```python
from build123d import *

# Parameters (mm, degrees)
F1_DEPTH = 12
F2_R     = 1.1
F3_DEPTH = 6.5
F4_R     = 2.5
F5_DEPTH = 25
F7_DEPTH = 32


with BuildPart() as f1:
    # F0 (on Right) → F1 (new body)
    with BuildSketch(Plane.YZ):
        Polygon((35.1, -0.075058), (-4.9, -0.075058), (-4.9, -25.075058), (0, -25.075058), (0, -10.075058), (3.1, -10.075058), (3.1, -25.075058), (35.1, -25.075058), align=None)
    extrude(amount=F1_DEPTH)

    # F2 (on face) → F3 (cut)
    with BuildSketch(Plane.YZ.offset(12)):
        Polygon((34.6, -2.396713), (18.6, -2.396713), (18.6, -22.896713), (34.6, -22.896713), (34.6, -13.396713), (38.479045, -13.396713), (38.479045, -2.396713), align=None)
        with Locations((26.6, -17.646713)):
            Circle(F2_R, mode=Mode.SUBTRACT)
        with Locations((26.6, -7.646713)):
            Circle(F2_R, mode=Mode.SUBTRACT)
    extrude(amount=-F3_DEPTH, mode=Mode.SUBTRACT)

    # F4 (on face) → F5 (cut)
    with BuildSketch(Plane(origin=(0, 18.6, 0), x_dir=(-1, 0, 0), z_dir=(0, 1, 0))):
        with Locations((-8.783709, -5.351877)):
            Circle(F4_R)
    extrude(amount=-F5_DEPTH, mode=Mode.SUBTRACT)

    # F6 (on face) → F7 (cut, through all)
    with BuildSketch(Plane(origin=(0, 35.1, 0), x_dir=(-1, 0, 0), z_dir=(0, 1, 0))):
        Polygon((1.341271, -20.075058), (-0.25, -20.075058), (-2.75, -22.575058), (-2.75, -25.075058), (1.341271, -25.075058), align=None)
    extrude(amount=-F7_DEPTH, mode=Mode.SUBTRACT)


solid = f1.part
```
Geometry check sheet. Reference: the model listing, model coordinates, mm. A direction names the side the tool comes from. Coordinates: 2 decimals unless noted, no trailing zeros. Loops run counter-clockwise (first coordinate to the right, second up) from the corner with the lowest first, then second, coordinate; pieces in that order, holes last. Notation, with made-up numbers: (29.5, 10.5) -> (80.5, 10.5) arc R33 ccw to (80.5, 46.5) -> close; hole circle Ø11 at (78, -5.5). An arc over 180 degrees is marked (long way). Put each result on its own line as item: value.
1) Gauge pin test, flat ends, axial feed: pin 1 Ø4 at (x, z) = (8.78, -5.35) entering from +Y; pin 2 Ø1.2 at (y, z) = (21.5, -24) entering from -X; pin 3 Ø1.6 at (x, y) = (4.5, 1.5) entering from -Z. Record the tip position at first contact, or that the pin passes through.
Result set:
pin 1: stops at y = 27.66
pin 2: stops at x = 2.75
pin 3: stops at z = -10.08
2) Release check for a two-part mould opening along X. For faces 4 (the cylindrical face through (6.4, 7, -4.6)), 5 (the flat face through (12, 10, -12)), 6 (the cylindrical face through (8.8, 27.19, -16.72)) record: released by +X, released by -X, zero draft, split by the parting line, or undercut.
Result set:
face 4: undercut
face 5: released by +X
face 6: zero draft
3) Cross-section at A-A on z = -15.5. Record the boundary of the cut face in (x, y), plus the area to 3 significant figures.
Result set:
outline: (0, -4.9) -> (12, -4.9) -> (12, 0) -> (0, 0) -> close; (0, 3.1) -> (12, 3.1) -> (12, 18.6) -> (5.5, 18.6) -> (5.5, 34.6) -> (12, 34.6) -> (12, 35.1) -> (0, 35.1) -> close
area: 339 mm^2
4) Tool access check on faces 1 (the flat face through (9, 34.6, -18)), 2 (the flat face through (6, 3.1, -17)), 3 (the flat face through (1.483, 19.324, -21.308)). Record the directions out of +Z, -Z, +X, -X, +Y, -Y that give a thin tool (end or side, any length) a straight path to the whole face; none if there is none.
Result set:
face 1: +X
face 2: -Z, +X, -X
face 3: -Z, -X, +Y
5) Cross-section at D-D on z = -12.5. Record the boundary of the cut face in (x, y).
Result set:
outline: (0, -4.9) -> (12, -4.9) -> (12, 0) -> (0, 0) -> close; (0, 3.1) -> (12, 3.1) -> (12, 18.6) -> (5.5, 18.6) -> (5.5, 35.1) -> (0, 35.1) -> close
6) Cross-section at C-C on y = 26.6. Record the boundary of the cut face in (x, z).
Result set:
outline: (0, -20.08) -> (0.25, -20.08) -> (2.75, -22.58) -> (2.75, -25.08) -> (12, -25.08) -> (12, -22.9) -> (5.5, -22.9) -> (5.5, -18.75) -> (12, -18.75) -> (12, -16.55) -> (5.5, -16.55) -> (5.5, -8.75) -> (12, -8.75) -> (12, -6.55) -> (5.5, -6.55) -> (5.5, -2.4) -> (12, -2.4) -> (12, -0.08) -> (0, -0.08) -> close
7) Cross-section at B-B on x = 9. Record the boundary of the cut face in (y, z), plus the area to 3 significant figures.
Result set:
outline: (-4.9, -25.08) -> (0, -25.08) -> (0, -10.08) -> (3.1, -10.08) -> (3.1, -25.08) -> (35.1, -25.08) -> (35.1, -13.4) -> (34.6, -13.4) -> (34.6, -22.9) -> (18.6, -22.9) -> (18.6, -7.84) -> (-4.9, -7.84) -> close; (-4.9, -2.86) -> (18.6, -2.86) -> (18.6, -2.4) -> (35.1, -2.4) -> (35.1, -0.08) -> (-4.9, -0.08) -> close; circle Ø2.2 at (26.6, -17.65); circle Ø2.2 at (26.6, -7.65)
area: 511 mm^2
8) Thickness scan on line 1 (Y direction, x = 8.75, z = -15.5); line 2 (Z direction, x = 6.5, y = 21); line 3 (Z direction, x = 10.25, y = 26.5). Record the ranges inside material, lowest first.
Result set:
line 1: y = -4.9 to 0, 3.1 to 18.6, 34.6 to 35.1
line 2: z = -25.08 to -22.9, -2.4 to -0.08
line 3: z = -25.08 to -22.9, -18.74 to -16.55, -8.74 to -6.55, -2.4 to -0.08
